from build123d import *

# Parameters (mm, degrees)
F0_W     = 70
F0_H     = 70
F1_DEPTH = 7
F3_DEPTH = 70
F4_R     = 3
F5_R     = 1
F6_R     = 1
F8_DEPTH = 7


with BuildPart() as f1:
    # F0 (on Top) → F1 (new body)
    with BuildSketch(Plane.XY):
        Rectangle(F0_W, F0_H)
    extrude(amount=F1_DEPTH)

    # F2 (on face) → F3 (cut, through all)
    with BuildSketch(Plane(origin=(-35, 0, 0), x_dir=(0, -1, 0), z_dir=(-1, 0, 0))):
        Polygon((31, 7), (21.4754591402, 7), (22.9629022167, 1.4487868654), (32.4874430764, 1.4487868654), align=None)
    extrude(amount=-F3_DEPTH, mode=Mode.SUBTRACT)

    # F4
    f4_edges = [f1.edges().sort_by_distance(p)[0] for p in [
        (0, -35, 7),
    ]]
    fillet(f4_edges, radius=F4_R)

    # F5
    f5_edges = [f1.edges().sort_by_distance(p)[0] for p in [
        (0, -35, 0),
    ]]
    fillet(f5_edges, radius=F5_R)

    # F6
    f6_edges = [f1.edges().sort_by_distance(p)[0] for p in [
        (0, -21.475459, 7),
        (0, -31, 7),
    ]]
    fillet(f6_edges, radius=F6_R)

    # F7 (on face) → F8 (cut, through all)
    with BuildSketch(Plane.XY.offset(7)):
        Polygon((-25, -19.4765049964), (25, -19.4765049964), (31.0781002045, 35), (26.0781002045, 35), (-25.1070436835, 35), (-30.1070436835, 35), align=None)
    extrude(amount=-F8_DEPTH, mode=Mode.SUBTRACT)


solid = f1.part
Work out the finished part from the listing and answer in its coordinate system (mm). A direction names the side the tool comes from. Give positions to 0.01 mm unless a question says otherwise; leave off trailing zeros. Loops run counter-clockwise (first coordinate to the right, second up) from the corner with the lowest first, then second, coordinate; pieces in that order, holes last. Notation, with made-up numbers: (42.25, 47) -> (47.25, 47) arc R23 cw to (47.25, 72) -> close; hole circle Ø9 at (27, 31.25). An arc over 180 degrees is marked (long way). Use a Markdown table: item, result. Add a question column.
1. Section C-C on y = 27.5 is taken. Determine the outline of the cut face in (x, z), and give its area (3 significant figures).
2. Determine the mould class of faces 1 (the flat face through (35, 7, 3)), 2 (the flat face through (-27.59, 8.14, 3.55)), 3 (the flat face through (0, -35, 2)) for opening direction X: released by +X, released by -X, zero draft, split by the parting line, or undercut.
3. For faces 4 (the flat face through (-0.49, -31.924, 3.553)), 5 (the cylindrical face through (0.49, -34.26, 5.97)), 6 (the flat face through (-0.49, -22.31, 3.89)), 7 (the flat face through (0, -19.477, 4)), determine the directions among +Z, -Z, +X, -X, +Y, -Y from which every point of the face is accessible in a straight line to the end or side of a thin tool.
4. Section A-A on y = -10 is taken. Determine the outline of the cut face in (x, z), and give its area (3 significant figures).
5. Section B-B on z = 2.5 is taken. Determine the outline of the cut face in (x, y).
6. Flat-ended cylindrical pins translate along their axes: pin 1 Ø4 at (x, z) = (-10.5, 3.5) entering from +Y; pin 2 Ø7.5 at (x, y) = (12.5, -27.5) entering from +Z. Find the tip coordinate at first contact, or state that the pin passes through.
7. Find the intervals of material crossed by probe 1 along Y at (x, z) = (-14, 4.25); probe 2 along X at (y, z) = (3.5, 4.5); probe 3 along Y at (x, z) = (12.5, 5.5), in increasing order.
Results below:
| question | item | result |
|---|---|---|
| 1 | outline | (-35, 0) -> (-29.4, 0) -> (-29.4, 7) -> (-35, 7) -> close; (30.24, 0) -> (35, 0) -> (35, 7) -> (30.24, 7) -> close |
| 1 | area | 72.5 mm^2 |
| 2 | face 1 | released by +X |
| 2 | face 2 | undercut |
| 2 | face 3 | zero draft |
| 3 | face 4 | +X, -X |
| 3 | face 5 | +Z, +X, -X, -Y |
| 3 | face 6 | +Z, +X, -X |
| 3 | face 7 | +Z, -Z, +Y |
| 4 | outline | (-35, 0) -> (-25.89, 0) -> (-25.89, 7) -> (-35, 7) -> close; (26.06, 0) -> (35, 0) -> (35, 7) -> (26.06, 7) -> close |
| 4 | area | 126 mm^2 |
| 5 | outline | (-35, -35) -> (35, -35) -> (35, -32.21) -> (-35, -32.21) -> close; (-35, -22.68) -> (35, -22.68) -> (35, 35) -> (31.08, 35) -> (25, -19.48) -> (-25, -19.48) -> (-30.11, 35) -> (-35, 35) -> close |
| 6 | pin 1 | stops at y = -19.48 |
| 6 | pin 2 | stops at z = 1.45 |
| 7 | probe 1 | y = -34.99 to -31.74, -22.21 to -19.48 |
| 7 | probe 2 | x = -35 to -27.15, 27.56 to 35 |
| 7 | probe 3 | y = -34.6 to -31.4, -21.88 to -19.48 |
